Could you check a few things on this drawing? It's one solid part, dimensions in mm from its lowest x, y, z. Round coordinates to 2 decimals unless told otherwise and drop trailing zeros. Loops run counter-clockwise (first coordinate to the right, second up) from the corner with the lowest first, then second, coordinate; pieces in that order, holes last.
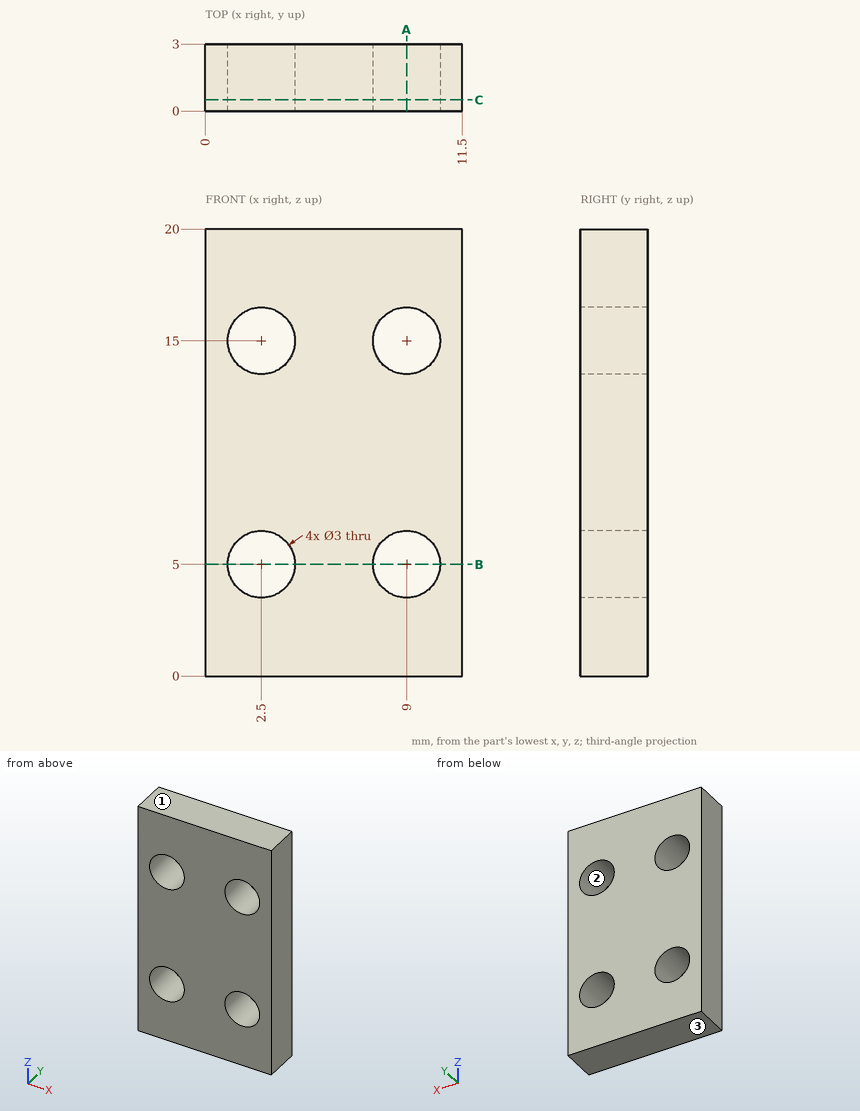
(1) Suppose I cut it at A-A (x = 9). Write out the boundary of the cut face in (y, z), then the cut area to 3 significant figures.
(2) Suppose I cut it at B-B (z = 5). Write out the boundary of the cut face in (x, y), then the cut area to 3 significant figures.
(3) Suppose I cut it at C-C (y = 0.5). Write out the boundary of the cut face in (x, z), then the cut area to 3 significant figures.
(4) For pin 1 (2.5 mm diameter, centred on x = 9, z = 15, fed in from +Y); pin 2 (1 mm diameter, centred on y = 1.5, z = 16, fed in from -X), each with a flat end and sliding along its axis, tell me the tip position at first contact or that it passes through.
(5) If I drill on line 1 (Z direction, x = 2.5, y = 2.1); line 2 (Z direction, x = 8, y = 1.9); line 3 (X direction, y = 1.75, z = 16.25), over which ranges is the centre line in solid material (lowest first)?
(6) We'd pull the mould along Z, two halves only. Please class the marked faces 1, 2 and 3: released by +Z, released by -Z, zero draft, split by the parting line, or undercut.
Check result:
1. outline: (0, 0) - (3, 0) - (3, 3.5) - (0, 3.5) - close; (0, 6.5) - (3, 6.5) - (3, 13.5) - (0, 13.5) - close; (0, 16.5) - (3, 16.5) - (3, 20) - (0, 20) - close
1. area: 42.0 mm2
2. outline: (0, 0) - (1, 0) - (1, 3) - (0, 3) - close; (4, 0) - (7.5, 0) - (7.5, 3) - (4, 3) - close; (10.5, 0) - (11.5, 0) - (11.5, 3) - (10.5, 3) - close
2. area: 16.5 mm2
3. outline: (0, 0) - (11.5, 0) - (11.5, 20) - (0, 20) - close; hole circle Ø3 at (2.5, 5); hole circle Ø3 at (2.5, 15); hole circle Ø3 at (9, 5); hole circle Ø3 at (9, 15)
3. area: 202 mm2
4. pin 1: passes through
4. pin 2: stops at x = 0
5. line 1: z = 0 to 3.5, 6.5 to 13.5, 16.5 to 20
5. line 2: z = 0 to 3.88, 6.12 to 13.88, 16.12 to 20
5. line 3: x = 0 to 1.67, 3.33 to 8.17, 9.83 to 11.5
6. face 1: released by +Z
6. face 2: undercut
6. face 3: released by -Z
